from build123d import *

# Parameters (mm, degrees)
BOSS_EXTRU_1_DEPTH      = 75
BOSS_EXTRU_2_START      = -70
BOSS_EXTRU_2_DEPTH      = 70
ENL_V_START             = -29
ENL_V_MAT_EXTRU_1_DEPTH = 29
CONG_1_R                = 30
CONG_2_R                = 10
ESQUISSE5_W             = 23
ESQUISSE5_H             = 42
ENL_V_MAT_EXTRU_2_DEPTH = 146.632261285


with BuildPart() as part:
    # Esquisse1 → Boss.-Extru.1 (new body)
    with BuildSketch(Plane(origin=(0, 11.1, 0), x_dir=(0, 0, 1), z_dir=(0, -1, 0))):
        with BuildLine():
            Line((-50.360184389, 1.826437931), (-53.360184389, 1.826437931))
            ThreePointArc((-53.360184389, 1.826437931), (-16.419058892, 36.821664014), (20.522066605, 1.826437931))
            Line((20.522066605, 1.826437931), (17.522066605, 1.826437931))
            ThreePointArc((17.522066605, 1.826437931), (-16.419058892, 33.826437931), (-50.360184389, 1.826437931))
        make_face()
    extrude(amount=BOSS_EXTRU_1_DEPTH)

    # Esquisse3 → Boss.-Extru.2 (add)
    with BuildSketch(Plane(origin=(0, -92.9, 0), x_dir=(-1, 0, 0), z_dir=(0, -1, 0)).offset(BOSS_EXTRU_2_START)):
        with BuildLine():
            Line((32, -1.84316049), (32, -59.576167192))
            Line((32, -59.576167192), (-12, -59.576167192))
            Line((-12, -59.576167192), (-12, -52.576167192))
            Line((-12, -52.576167192), (12, -52.576167192))
            Line((12, -52.576167192), (12, -18.515896948))
            ThreePointArc((12, -18.515896948), (23.515293751, -11.997219241), (32, -1.84316049))
        make_face()
    extrude(amount=BOSS_EXTRU_2_DEPTH)

    # Esquisse4 → Enlèv. mat.-Extru.1 (cut)
    with BuildSketch(Plane.XZ.offset(92.9).offset(ENL_V_START)):
        with BuildLine():
            Line((-12, 18.515896948), (-12, 52.576167192))
            Line((-12, 52.576167192), (-32, 52.576167192))
            Line((-32, 52.576167192), (-32, 1.84316049))
            ThreePointArc((-32, 1.84316049), (-23.515293751, 11.997219241), (-12, 18.515896948))
        make_face()
    extrude(amount=ENL_V_MAT_EXTRU_1_DEPTH, mode=Mode.SUBTRACT)

    # Congé1
    cong_1_edges = [part.edges().sort_by_distance(p)[0] for p in [
        (-32, -43.4, 1.84316049),
    ]]
    fillet(cong_1_edges, radius=CONG_1_R)

    # Congé2
    # the kernel refuses this fillet: 10 mm, written as the material it adds along each edge
    with BuildSketch(Plane(origin=(-12, -22.9, 18.515896948), x_dir=(0, 0, 1), z_dir=(0, -1, 0))) as cong_2_piece_1_section:
        with BuildLine():
            CenterArc((12.004663354, -10), CONG_2_R, 90, 90.994487339)
            Line((2.006169657, -10.173562069), (1.806199783, -10.177033311))
            ThreePointArc((1.806199783, -10.177033311), (1.165077614, -5.054836961), (-0.188861967, -0.06581153))
            Line((-0.188861967, -0.06581153), (0, 0.2))
            Line((0, 0.2), (12.004663354, 0.2))
            Line((12.004663354, 0.2), (12.004663354, 0))
        make_face()
    cong_2_piece_1 = extrude(amount=41, mode=Mode.PRIVATE)
    cong_2_piece_1 = split(cong_2_piece_1, bisect_by=Plane(origin=(-1.826437931, -43.4, 22.039675227), z_dir=(-1, 0, 0)), keep=Keep.TOP, mode=Mode.PRIVATE)
    add(cong_2_piece_1)

    # Esquisse5 → Enlèv. mat.-Extru.2 (cut, through all)
    with BuildSketch(Plane(origin=(0, 0, 52.576167192), x_dir=(-1, 0, 0), z_dir=(0, 0, -1))):
        with Locations((-0.5, -63.4)):
            Rectangle(ESQUISSE5_W, ESQUISSE5_H)
        with BuildLine():
            Line((-6, -36.25), (-4, -36.25))
            ThreePointArc((-4, -36.25), (-1.75, -38.5), (-4, -40.75))
            Line((-4, -40.75), (-6, -40.75))
            ThreePointArc((-6, -40.75), (-8.25, -38.5), (-6, -36.25))
        make_face()
        with BuildLine():
            Line((4, -36.25), (6, -36.25))
            ThreePointArc((6, -36.25), (8.25, -38.5), (6, -40.75))
            Line((6, -40.75), (4, -40.75))
            ThreePointArc((4, -40.75), (1.75, -38.5), (4, -36.25))
        make_face()
        with BuildLine():
            Line((-6, -86.25), (-4, -86.25))
            ThreePointArc((-4, -86.25), (-1.75, -88.5), (-4, -90.75))
            Line((-4, -90.75), (-6, -90.75))
            ThreePointArc((-6, -90.75), (-8.25, -88.5), (-6, -86.25))
        make_face()
        with BuildLine():
            Line((4, -86.25), (6, -86.25))
            ThreePointArc((6, -86.25), (8.25, -88.5), (6, -90.75))
            Line((6, -90.75), (4, -90.75))
            ThreePointArc((4, -90.75), (1.75, -88.5), (4, -86.25))
        make_face()
    extrude(amount=-ENL_V_MAT_EXTRU_2_DEPTH, mode=Mode.SUBTRACT)


solid = part.part
Part model, mm, in its own coordinate system. A direction names the side the tool comes from. Round coordinates to 2 decimals unless told otherwise and drop trailing zeros. Write each loop counter-clockwise with the first axis right and the second up, starting at its lowest first coordinate (ties: lowest second). Pieces come first, ordered by that corner, then holes. Notation, with made-up numbers: M 27.25,69 L 51.25,69 A19 cw 51.25,98 Z; hole C 77.25,46 d10. An arc over 180 degrees is marked long. Return JSON: item names as keys, results as strings. Group by question number.
(1) Which spindle directions (+Z, -Z, +X, -X, +Y, -Y) get a long thin tool onto all of the face, cutting with end or side? Do faces 1 (the face through (-23, -63.9, 19)), 2 (the face through (-8.25, -38.45, 56.03)), 3 (the face through (-34.473, -25.875, -29.392)). Say none if no direction does.
(2) Saw through at C-C on y = -56.5. Write the cut outline in (x, z).
(3) Two-plate mould, pull along X, no slides. Class faces 4 (the face through (8.25, -88.55, 56.03)), 5 (the face through (-1.75, -88.55, 56.03)), 6 (the face through (-15, -65, 52.576)), 7 (the face through (-12, -43, 42)): +X half, -X half, draft (parallel to the pull), parting line (faces both ways), or undercut.
(4) Saw through at D-D on z = -43. Write the cut outline in (x, y), then the cut area to 3 significant figures.
(5) Saw through at B-B on x = -16. Write the cut outline in (y, z).
(6) Drill centre lines: probe 1 along Y at (x, z) = (-17, 55.5); probe 2 along Z at (x, y) = (-16, -50); probe 3 along Z at (x, y) = (-24, -39). Where is each one in solid material? Low to high.
(7) Pin check, flat tips, straight feed: pin 1 Ø10.5 at (x, z) = (-16.5, 20) entering from -Y; pin 2 Ø6 at (x, z) = (-27.5, -26.5) entering from -Y; pin 3 Ø1.6 at (x, z) = (5, 58) entering from +Y; pin 4 Ø8 at (x, y) = (-2.5, -57) entering from +Z. Stop position of each tip, or through.
(8) Saw through at A-A on y = -88.5. Write the cut outline in (x, z), then the cut area to 3 significant figures.
Returned:
{
 "1": {"face 1": "-Z, +X, -X, -Y", "face 2": "+Z", "face 3": "-X, +Y"},
 "2": {"outline": "M -34.16,-2.64 A37 ccw -1.83,-53.36 L -1.83,-50.36 A34 cw -1.83,17.52 L -1.83,20.52 A10 cw -12,30.52 L -12,52.58 L -11,52.58 L -11,59.58 L -32,59.58 L -32,8.54 A30 cw Z"},
 "3": {"face 4": "undercut", "face 5": "undercut", "face 6": "draft", "face 7": "+X half"},
 "4": {"outline": "M -25.56,-63.9 L -21.03,-63.9 L -21.03,11.1 L -25.56,11.1 Z", "area": "340 mm²"},
 "5": {"outline": "M -92.9,52.58 L -63.9,52.58 L -63.9,13.49 L 11.1,13.49 L 11.1,16.85 L -22.9,16.85 L -22.9,59.58 L -92.9,59.58 Z; M -63.9,-49.69 L 11.1,-49.69 L 11.1,-46.33 L -63.9,-46.33 Z"},
 "6": {"probe 1": "-92.9 to -22.9", "probe 2": "-49.69 to -46.33, 13.49 to 59.58", "probe 3": "-44.42 to -40.33, 7.49 to 59.58"},
 "7": {"pin 1": "y = -63.9", "pin 2": "through", "pin 3": "y = -22.9", "pin 4": "z = 21.59"},
 "8": {"outline": "M -32,52.58 L -8.25,52.58 L -8.25,59.58 L -32,59.58 Z; M -1.75,52.58 L 1.75,52.58 L 1.75,59.58 L -1.75,59.58 Z; M 8.25,52.58 L 12,52.58 L 12,59.58 L 8.25,59.58 Z", "area": "217 mm²"}
}
